Geometry: final body of the model. Coordinates: model frame, mm. Coordinates: 2 decimals unless noted, no trailing zeros. Write each loop counter-clockwise with the first axis right and the second up, starting at its lowest first coordinate (ties: lowest second). Pieces come first, ordered by that corner, then holes. Notation, with made-up numbers: M 33.5,47.25 L 78.5,47.25 A12 ccw 78.5,59.25 Z; hole C 29.5,23.25 d5. An arc over 180 degrees is marked long. Write item = value, one per line. Start each with the question number.
Item 1: Section C-C on x = -154.5. Output: boundary loops of the cut face in (y, z), plus the area to 3 significant figures.
Item 2: Ray query, L1, parallel to X at y = -165, z = 1.4; L2, parallel to Y at x = -110, z = 0.15; L3, parallel to Y at x = -206.5, z = 1.2. Return the intervals inside material, ascending. Write a range as [from, to].
Item 3: First-contact query: pin 1 Ø4 at (x, y) = (-12.68, -25) entering from +Z; pin 2 Ø1 at (x, z) = (-187, 0.5) entering from +Y. Flat tips, straight axial feed; report the tip coordinate or a pass-through.
Item 4: Section A-A on z = 1.45. Output: boundary loops of the cut face in (x, y).
Item 5: Section B-B on y = -59.5. Output: boundary loops of the cut face in (x, z), plus the area to 3 significant figures.
from build123d import *

# Parameters (mm, degrees)
EXTRUDE_1_DEPTH     = 2
SKETCH_4_R          = 1.55
CUT_EXTRUDE_1_DEPTH = 2


with BuildPart() as part:
    # Эскиз3 → Бобышка-Вытянуть1 (new body)
    with BuildSketch(Plane.XY):
        Polygon((0, -209.31740407), (-101.035924752, -267.65564884), (-282.318078778, -163.01074319), (0, 0), align=None)
    extrude(amount=EXTRUDE_1_DEPTH)

    # Эскиз4 → Вырез-Вытянуть1 (cut)
    with BuildSketch(Plane(origin=(0, 0, 0), x_dir=(-1, 0, 0), z_dir=(0, 0, -1))):
        with Locations((254.324370014, -164.525982342)):
            Circle(SKETCH_4_R)
        with Locations((103.664201466, -251.49438366)):
            Circle(SKETCH_4_R)
        with Locations((12.682716025, -198.961582281)):
            Circle(SKETCH_4_R)
        with Locations((12.682716025, -25.001847817)):
            Circle(SKETCH_4_R)
    extrude(amount=-CUT_EXTRUDE_1_DEPTH, mode=Mode.SUBTRACT)


solid = part.part
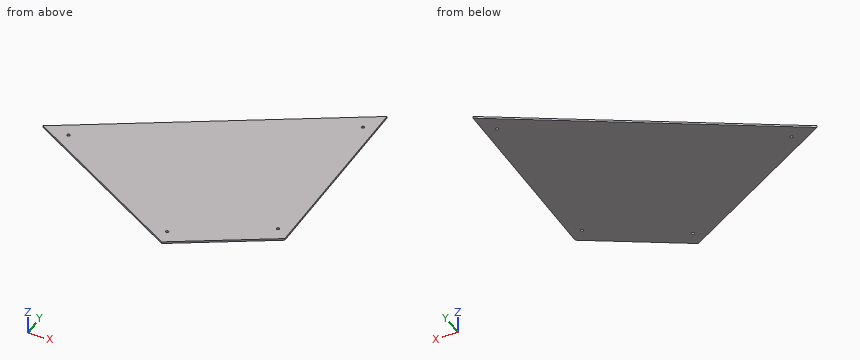
Responses:
q1.outline = M -236.79,0 L -89.21,0 L -89.21,2 L -236.79,2 Z
q1.area = 295 mm²
q2.L1 = [-278.87, -255.8], [-252.85, 0]
q2.L2 = [-262.48, -63.51]
q2.L3 = [-206.78, -119.23]
q3.pin_1 = 2
q3.pin_2 = -107.69
q4.outline = M -282.32,-163.01 L -101.04,-267.66 L 0,-209.32 L 0,0 Z; hole C -254.32,-164.53 d3.1; hole C -103.66,-251.49 d3.1; hole C -12.68,-198.96 d3.1; hole C -12.68,-25 d3.1
q5.outline = M -103.05,0 L 0,0 L 0,2 L -103.05,2 Z
q5.area = 206 mm²
